from build123d import *

# Parameters (mm, degrees)
CROQUIS1_W              = 202
CROQUIS1_H              = 30
CROQUIS1_R              = 5
SALIENTE_EXTRUIR1_DEPTH = 60
CROQUIS2_W              = 192
CROQUIS2_H              = 50
CORTAR_EXTRUIR1_DEPTH   = 169.836501235


with BuildPart() as part:
    # Croquis1 → Saliente-Extruir1 (new body)
    with BuildSketch(Plane(origin=(0, 0, 0), x_dir=(1, 0, 0), z_dir=(0, 1, 0))):
        with Locations((53.937936443, 4.098360656)):
            Rectangle(CROQUIS1_W, CROQUIS1_H)
        with Locations(Location((-37.062063557, 4.098360656, 0), (0, 0, 270))):
            Circle(CROQUIS1_R, mode=Mode.SUBTRACT)
        with Locations(Location((144.937936443, 4.098360656, 0), (0, 0, 270))):
            Circle(CROQUIS1_R, mode=Mode.SUBTRACT)
    extrude(amount=SALIENTE_EXTRUIR1_DEPTH)

    # Croquis2 → Cortar-Extruir1 (cut, through all)
    with BuildSketch(Plane.XY.offset(10.901639344)):
        with Locations((53.937936443, 30)):
            Rectangle(CROQUIS2_W, CROQUIS2_H)
    extrude(amount=-CORTAR_EXTRUIR1_DEPTH, mode=Mode.SUBTRACT)


solid = part.part
For this review, take the finished solid that the model builds, in its own axes (mm). A direction names the side the tool comes from. Give positions to 0.01 mm unless a question says otherwise; leave off trailing zeros. Order: outer loops, then holes, each group sorted by start corner. A loop starts at its lowest first (then second) coordinate and runs counter-clockwise, first axis right, second up. Notation, with made-up numbers: (66.25, 34) - (83.25, 34) arc R17 cw to (83.25, 59) - close; hole circle Ø9 at (-26, 89). An arc over 180 degrees is marked (long way). Answer as a JSON object with one key per item and string values. Group by question number.
Item 1: Clearance check with a flat-ended pin moving along its axis: pin 1 Ø8 at (x, z) = (144.94, -4.1) entering from -Y. State where the tip first meets the part, or that it passes through.
Item 2: Take a section at C-C on z = -16.25. Give the boundary of the cut face in (x, y), and give its area (3 significant figures).
Item 3: Take a section at B-B on x = 107. Give the boundary of the cut face in (y, z), and give its area (3 significant figures).
Item 4: Wall thickness on line 1 along X through (y, z) = (11.5, -14.75); line 2 along X through (y, z) = (4.5, -3.25); line 3 along Y through (x, z) = (1, -3.5): over which ranges is each line inside the solid? List them lowest first.
Item 5: Draft analysis for pull direction Z (two halves, no side actions). For faces 3 (the cylindrical face through (-41.943, 57.465, -5.182)), 4 (the flat face through (53, 5, -4)), 5 (the flat face through (46, 57, 10.902)), state which applies: pulls with the +Z half, pulls with the -Z half, needs draft (parallel to the pull), parting line crosses it, or undercut.
Item 6: Take a section at A-A on y = 39. Give the boundary of the cut face in (x, z).
Item 7: Machinability: for faces 1 (the flat face through (53, 60, -4)), 2 (the flat face through (149.938, 30, -4)), which of the approach directions +Z, -Z, +X, -X, +Y, -Y give a long, thin tool a straight path to every point of the face, cutting with its end or side? Answer none if there is none.
Reported:
{
 "1": {"pin 1": "through"},
 "2": {"outline": "(-47.06, 0) - (154.94, 0) - (154.94, 60) - (-47.06, 60) - close; hole (-42.06, 5) - (149.94, 5) - (149.94, 55) - (-42.06, 55) - close", "area": "2,520 mm^2"},
 "3": {"outline": "(0, -19.1) - (5, -19.1) - (5, 10.9) - (0, 10.9) - close; (55, -19.1) - (60, -19.1) - (60, 10.9) - (55, 10.9) - close", "area": "300 mm^2"},
 "4": {"line 1": "-47.06 to -42.06, 149.94 to 154.94", "line 2": "-47.06 to -41.99, -32.13 to 140.01, 149.87 to 154.94", "line 3": "0 to 5, 55 to 60"},
 "5": {"face 3": "undercut", "face 4": "needs draft", "face 5": "pulls with the +Z half"},
 "6": {"outline": "(-47.06, -19.1) - (-42.06, -19.1) - (-42.06, 10.9) - (-47.06, 10.9) - close; (149.94, -19.1) - (154.94, -19.1) - (154.94, 10.9) - (149.94, 10.9) - close"},
 "7": {"face 1": "+Z, -Z, +X, -X, +Y", "face 2": "+Z, -Z"}
}
